```python
from build123d import *

# Parameters (mm, degrees)
F1_DEPTH = 3.81
F3_DEPTH = 25.4
F4_W     = 5.08
F4_H     = 7.62
F5_DEPTH = 50.8


with BuildPart() as f1:
    # F0 (on Top) → F1 (new body)
    with BuildSketch(Plane.XY):
        Polygon((-29.753983, 4.73037), (-44.993983, 4.73037), (-44.993983, 0.92037), (-38.643983, 0.92037), (-38.643983, -6.69963), (-44.993983, -6.69963), (-44.993983, -10.50963), (-29.753983, -10.50963), align=None)
    extrude(amount=F1_DEPTH)

    # F2 (on face) → F3 (join)
    with BuildSketch(Plane(origin=(0, 0, 0), x_dir=(1, 0, 0), z_dir=(0, 0, -1))):
        Polygon((-29.753983, 10.50963), (-38.643983, 10.50963), (-38.643983, 6.69963), (-38.643983, -0.92037), (-38.643983, -4.73037), (-29.753983, -4.73037), align=None)
    extrude(amount=F3_DEPTH)

    # F4 (on face) → F5 (cut)
    with BuildSketch(Plane(origin=(0, 0, -25.4), x_dir=(1, 0, 0), z_dir=(0, 0, -1))):
        with Locations((-36.103983, 2.88963)):
            Rectangle(F4_W, F4_H)
    extrude(amount=-F5_DEPTH, mode=Mode.SUBTRACT)


solid = f1.part
```
CAD build for the part. Positions are in the model's coordinates, mm. A direction names the side the tool comes from. Round coordinates to 2 decimals unless told otherwise and drop trailing zeros. Order: outer loops, then holes, each group sorted by start corner. A loop starts at its lowest first (then second) coordinate and runs counter-clockwise, first axis right, second up.
Item 1: Saw through at B-B on y = 2.25. Write the cut outline in (x, z), then the cut area to 3 significant figures.
Item 2: Tool access for faces 1 (the face through (-33, -3, -25.4)), 2 (the face through (-37, 0.92, -11)), 3 (the face through (-38.644, 3, -13)): list every direction of +Z, -Z, +X, -X, +Y, -Y with a clear straight run to the whole face (end or side of a thin tool).
Item 3: Mould opens along Y. For faces 4 (the face through (-37, -6.7, -11)), 5 (the face through (-34, -10.51, -11)), 6 (the face through (-44.994, 3, 2)) say: pulls with the +Y half, pulls with the -Y half, needs draft (parallel to the pull), parting line crosses it, or undercut.
Item 4: Saw through at D-D on x = -41.75. Write the cut outline in (y, z).
Item 5: Probe line 1 along Y through (x, z) = (-42.5, 2); line 2 along X through (y, z) = (-8.25, -17.5); line 3 along X through (y, z) = (-4, -15.75). List the from-to ranges inside material, lowest first.
Item 6: Saw through at C-C on z = -16. Write the cut outline in (x, y), then the cut area to 3 significant figures.
Item 7: Saw through at A-A on x = -34.5. Write the cut outline in (y, z), then the cut area to 3 significant figures.
Item 8: Pin check, flat tips, straight feed: pin 1 (6 mm diameter, centred on y = -3, z = -8, fed in from -X); pin 2 (3.5 mm diameter, centred on x = -41, z = -15.5, fed in from +Y); pin 3 (8 mm diameter, centred on x = -39, z = -22.5, fed in from -Y); pin 4 (4 mm diameter, centred on y = -8, z = -16, fed in from -X). Stop position of each tip, or through.
Reported:
1. outline: (-44.99, 0) - (-38.64, 0) - (-38.64, -25.4) - (-29.75, -25.4) - (-29.75, 3.81) - (-44.99, 3.81) - close
1. area: 284 mm2
2. face 1: -Z, +X, -X, +Y, -Y
2. face 2: +Z, -Z, -X
2. face 3: -Z, -X, +Y, -Y
3. face 4: undercut
3. face 5: pulls with the -Y half
3. face 6: needs draft
4. outline: (-10.51, 0) - (-6.7, 0) - (-6.7, 3.81) - (-10.51, 3.81) - close; (0.92, 0) - (4.73, 0) - (4.73, 3.81) - (0.92, 3.81) - close
5. line 1: y = -10.51 to -6.7, 0.92 to 4.73
5. line 2: x = -38.64 to -29.75
5. line 3: x = -33.56 to -29.75
6. outline: (-38.64, -10.51) - (-29.75, -10.51) - (-29.75, 4.73) - (-38.64, 4.73) - (-38.64, 0.92) - (-33.56, 0.92) - (-33.56, -6.7) - (-38.64, -6.7) - close
6. area: 96.8 mm2
7. outline: (-10.51, -25.4) - (-6.7, -25.4) - (-6.7, 3.81) - (-10.51, 3.81) - close; (0.92, -25.4) - (4.73, -25.4) - (4.73, 3.81) - (0.92, 3.81) - close
7. area: 223 mm2
8. pin 1: stops at x = -33.56
8. pin 2: passes through
8. pin 3: stops at y = -10.51
8. pin 4: stops at x = -38.64
